```python
from build123d import *

# Parameters (mm, degrees)
BOSS_EXTRUDE4_DEPTH = 1.59
SKETCH5_W           = 7.725
SKETCH5_H           = 25
SKETCH5_R           = 1.47
BOSS_EXTRUDE5_DEPTH = 3.18
SKETCH7_R           = 1.47
CUT_EXTRUDE1_DEPTH  = 52.250588065


with BuildPart() as part:
    # Sketch2 → Boss-Extrude4 (new, symmetric)
    with BuildSketch(Plane.XY):
        Polygon((-28, -6.144451952), (28, -6.144451952), (28, 12.576257704), (28, 34.894451952), (20.275, 34.894451952), (20.275, 6.144451952), (-20.275, 6.144451952), (-20.275, 34.894451952), (-28, 34.894451952), (-28, 2.372923503), align=None)
    extrude(amount=BOSS_EXTRUDE4_DEPTH, both=True)

    # Sketch5 → Boss-Extrude5 (add)
    with BuildSketch(Plane(origin=(0, 34.894451952, 0), x_dir=(1, 0, 0), z_dir=(0, 1, 0))):
        with Locations((24.1375, 14.09)):
            Rectangle(SKETCH5_W, SKETCH5_H)
        with Locations(Location((24.975, 8.17, 0), (0, 0, 270))):
            Circle(SKETCH5_R, mode=Mode.SUBTRACT)
        with Locations(Location((24.975, 18.33, 0), (0, 0, 270))):
            Circle(SKETCH5_R, mode=Mode.SUBTRACT)
    boss_extrude5 = extrude(amount=-BOSS_EXTRUDE5_DEPTH)

    # Mirror1: Boss-Extrude5 across plane
    add(boss_extrude5.mirror(Plane(origin=(0, 0, 0), x_dir=(0, 0, 1), z_dir=(1, 0, 0))))

    # Sketch7 → Cut-Extrude1 (cut, through all)
    with BuildSketch(Plane(origin=(0, 0, -1.59), x_dir=(-1, 0, 0), z_dir=(0, 0, -1))):
        Circle(SKETCH7_R)
        with Locations((24.1375, 13.855548048)):
            Circle(SKETCH7_R)
        with Locations((-24.1375, 13.855548048)):
            Circle(SKETCH7_R)
    extrude(amount=-CUT_EXTRUDE1_DEPTH, mode=Mode.SUBTRACT)


solid = part.part
```
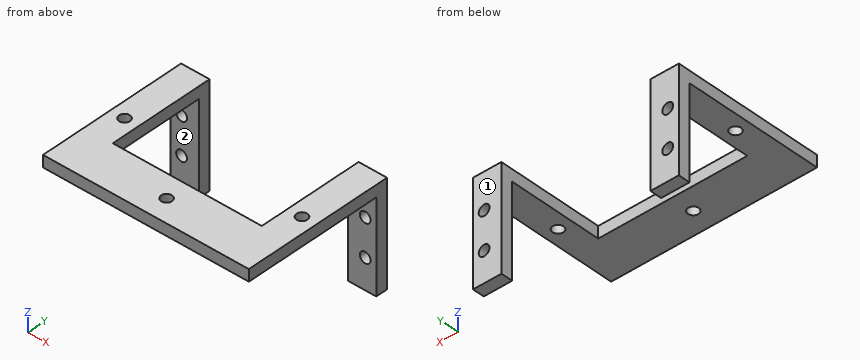
Could you check a few things on this model? Use its own coordinates, in mm. Face numbers are marked on the shaded views. A direction names the side the tool comes from. Coordinates: 2 decimals unless noted, no trailing zeros. Write each loop counter-clockwise with the first axis right and the second up, starting at its lowest first coordinate (ties: lowest second). Pieces come first, ordered by that corner, then holes. Notation, with made-up numbers: (13, -38.5) -> (18, -38.5) arc R24 ccw to (18, -27.5) -> close; hole circle Ø9 at (75.5, 12.5). An arc over 180 degrees is marked (long way). One line per question, with ' | ' between items. Start each with the question number.
1. If we section it at C-C (x = 0): Please give me the cut outline in (y, z), and give its area (3 significant figures).
2. For the marked faces 1 and 2, which set-ups out of +Z, -Z, +X, -X, +Y, -Y let a thin tool reach every point of the face, with its end or its side?
3. Please list where these lines run through material, in increasing order: line 1 along X through (y, z) = (33.05, -8.17) (3 decimals); line 2 along Z through (x, y) = (17.5, 0.5); line 3 along Y through (x, z) = (23, -2.25).
4. If we section it at A-A (y = 21): Please give me the cut outline in (x, z) (3 decimals), and give its area (3 significant figures).
5. If we section it at B-B (z = -18.33): Please give me the cut outline in (x, y) (3 decimals).
6. Will these pins go through, and if not, where does the flat tip stop? P1, Ø2.5, axis at x = -25, z = -16.5, coming from the -Y side; P2, Ø2.5, axis at x = 24.14, y = 13.86, coming from the -Z side; P3, Ø2.5, axis at x = 4.5, z = -1, coming from the +Y side.
7. If we section it at D-D (y = 32.5): Please give me the cut outline in (x, z) (3 decimals), and give its area (3 significant figures).
Return value:
1) outline: (-6.14, -1.59) -> (-1.47, -1.59) -> (-1.47, 1.59) -> (-6.14, 1.59) -> close; (1.47, -1.59) -> (6.14, -1.59) -> (6.14, 1.59) -> (1.47, 1.59) -> close | area: 29.7 mm²
2) face 1: +Z, -Z, +X, -X, +Y | face 2: -Z, +X, -X, -Y
3) line 1: x = -28 to -26.445, -23.505 to -20.275, 20.275 to 23.505, 26.445 to 28 | line 2: z = -1.59 to 1.59 | line 3: y = 31.71 to 34.89
4) outline: (-28, -1.59) -> (-20.275, -1.59) -> (-20.275, 1.59) -> (-28, 1.59) -> close; (20.275, -1.59) -> (28, -1.59) -> (28, 1.59) -> (20.275, 1.59) -> close | area: 49.1 mm²
5) outline: (-28, 31.714) -> (-26.445, 31.714) -> (-26.445, 34.894) -> (-28, 34.894) -> close; (-23.505, 31.714) -> (-20.275, 31.714) -> (-20.275, 34.894) -> (-23.505, 34.894) -> close; (20.275, 31.714) -> (23.505, 31.714) -> (23.505, 34.894) -> (20.275, 34.894) -> close; (26.445, 31.714) -> (28, 31.714) -> (28, 34.894) -> (26.445, 34.894) -> close
6) P1: stops at y = 31.71 | P2: passes through | P3: stops at y = 6.14
7) outline: (-28, -26.59) -> (-20.275, -26.59) -> (-20.275, 1.59) -> (-28, 1.59) -> close; (20.275, -26.59) -> (28, -26.59) -> (28, 1.59) -> (20.275, 1.59) -> close; hole circle Ø2.94 at (-24.975, -18.33); hole circle Ø2.94 at (-24.975, -8.17); hole circle Ø2.94 at (24.975, -18.33); hole circle Ø2.94 at (24.975, -8.17) | area: 408 mm²
